Check sheet for the modelled part. Datum: model origin and axes. Units: mm. A direction names the side the tool comes from. Give positions to 0.01 mm unless a question says otherwise; leave off trailing zeros. Write each loop counter-clockwise with the first axis right and the second up, starting at its lowest first coordinate (ties: lowest second). Pieces come first, ordered by that corner, then holes. Notation, with made-up numbers: M 14,47 L 33,47 A11 ccw 33,59 Z; hole C -22,26.25 d10. An arc over 180 degrees is marked long. One line per item, written item: value. Start each with the question number.
Autodesk Inventor part; units mm, degrees
ref_plane "YZ Plane" through (0, 0, 0) normal (1, 0, 0) x (0, 1, 0)
ref_plane "XZ Plane" through (0, 0, 0) normal (0, 1, 0) x (-1, 0, 0)
ref_plane "XY Plane" through (0, 0, 0) normal (0, 0, 1) x (1, 0, 0)
sketch "Boceto1" plane through (0, 0, 0) normal (0, 0, 1) x (1, 0, 0)
  line L0 (3, -11.4) -> (3, -5.5)
  line L1 (3, -5.5) -> (-2.2, -5.5)
  arc A0 (-5.5, -2.2) -> (-2.2, -5.5) centre (-2.2, -2.2) ccw
  line L2 (-5.5, -2.2) -> (-5.5, 2.2)
  arc A1 (-2.2, 5.5) -> (-5.5, 2.2) centre (-2.2, 2.2) ccw
  line L3 (-2.2, 5.5) -> (3, 5.5)
  line L4 (3, 5.5) -> (3, 11.4)
  line L5 (3, 3) -> (-2.2, 3)
  arc A2 (-2.2, 3) -> (-3, 2.2) centre (-2.2, 2.2) ccw
  line L6 (-3, 2.2) -> (-3, -2.2)
  arc A3 (-3, -2.2) -> (-2.2, -3) centre (-2.2, -2.2) ccw
  line L7 (-2.2, -3) -> (3, -3)
  line L8 (3, -3) -> (3, 3)
  line L9 (-2.2, 3.25) -> (3.25, 3.25)
  line L10 (3.25, 3.25) -> (3.25, -3.25)
  line L11 (3.25, -3.25) -> (-2.2, -3.25)
  arc A4 (-3.25, -2.2) -> (-2.2, -3.25) centre (-2.2, -2.2) ccw
  line L12 (-3.25, -2.2) -> (-3.25, 2.2)
  arc A5 (-2.2, 3.25) -> (-3.25, 2.2) centre (-2.2, 2.2) ccw
  line L13 (-2.2, 5) -> (5, 5)
  line L14 (5, 5) -> (5, -5)
  line L15 (5, -5) -> (-2.2, -5)
  arc A6 (-5, -2.2) -> (-2.2, -5) centre (-2.2, -2.2) ccw
  line L16 (-5, -2.2) -> (-5, 2.2)
  arc A7 (-2.2, 5) -> (-5, 2.2) centre (-2.2, 2.2) ccw
  line L17 (5, 0) -> (23, 0)
  line L18 (5, 5) -> (6.5, 5)
  line L19 (8.8007, 5) -> (8.0007, 5)
  line L20 (8.0007, 5) -> (8.0007, -5)
  line L21 (8.0007, -5) -> (8.8007, -5)
  line L22 (8.8007, -5) -> (8.8007, 5)
  line L23 (8.8007, -5) -> (10.3007, -5)
  line L24 (12.6007, -5) -> (11.8007, -5)
  line L25 (11.8007, -5) -> (11.8007, 5)
  line L26 (11.8007, 5) -> (12.6007, 5)
  line L27 (12.6007, 5) -> (12.6007, -5)
  arc A8 (8.8007, -5) -> (11.8007, -5) centre (10.3007, -5) ccw
  arc A9 (8.0007, -5) -> (12.6007, -5) centre (10.3007, -5) ccw
  arc A10 (8.0007, 5) -> (4.9993, 5) centre (6.5, 5) ccw
  arc A11 (8.8007, 5) -> (4.1993, 5) centre (6.5, 5) ccw
  line L28 (16.4021, 5) -> (15.6021, 5)
  line L29 (15.6021, 5) -> (15.6021, -5)
  line L30 (15.6021, -5) -> (16.4021, -5)
  line L31 (16.4021, -5) -> (16.4021, 5)
  line L32 (20.2021, -5) -> (19.4021, -5)
  line L33 (19.4021, -5) -> (19.4021, 5)
  line L34 (19.4021, 5) -> (20.2021, 5)
  line L35 (20.2021, 5) -> (20.2021, -5)
  arc A12 (16.4021, -5) -> (19.4021, -5) centre (17.9021, -5) ccw
  arc A13 (15.6021, -5) -> (20.2021, -5) centre (17.9021, -5) ccw
  arc A14 (15.6021, 5) -> (12.6007, 5) centre (14.1014, 5) ccw
  arc A15 (16.4021, 5) -> (11.8007, 5) centre (14.1014, 5) ccw
  line L36 (24.0036, 5) -> (23.2036, 5)
  line L37 (23.2036, 5) -> (23.2036, -0.2574)
  line L38 (23.2036, -5) -> (24.0036, -5)
  line L39 (24.0036, -1.1409) -> (24.0036, 5)
  arc A16 (23.2036, 5) -> (20.2021, 5) centre (21.7028, 5) ccw
  arc A17 (24.0036, 5) -> (19.4021, 5) centre (21.7028, 5) ccw
  arc A18 (26.3756, 8.5) -> (24.3756, 0) centre (41.5966, 0.4333) ccw
  circle A19 centre (24.3756, 0) radius 1.2
  arc A20 (27.4359, 7.9381) -> (25.5752, 0.0302) centre (41.5966, 0.4333) ccw
  line L40 (25.6, 8.5) -> (25.9736, 8.302)
  arc A21 (27.4359, 7.9381) -> (26.3756, 8.5) centre (26.9058, 8.219) ccw
  arc A22 (24.3756, 0) -> (26.3756, -8.5) centre (41.5966, -0.4333) ccw
  arc A23 (26.3756, -8.5) -> (27.4359, -7.9381) centre (26.9058, -8.219) ccw
  line L41 (26.7492, -8.302) -> (27.4359, -7.9381)
  arc A24 (25.5752, -0.0302) -> (27.4359, -7.9381) centre (41.5966, -0.4333) ccw
  line L42 (23.2036, 0) -> (24.0036, 0)
  point P0 (0, 0)
  point P1 (5, -5)
  point P2 (4.2, -5)
  point P3 (3.8, 5)
  point P4 (25.5036, -5)
  point P5 (22.4, 0)
  point P6 (24.3872, 1.1999)
  point P7 (24.0036, 1.1409)
  point P8 (23.2036, 0.2574)
  point P9 (24.3872, -1.1999)
  point P10 (25.5752, -0.0302)
  point P11 (25.5752, 0.0302)
  dimension "d1" = 0.25
  dimension "d2" = 2
  dimension "d42" = 18
  dimension "d43" = 1.5
  dimension "d45" = 0.8
  dimension "d46" = 10
  dimension "d47" = 1.5
  dimension "d48" = 0.8
  dimension "d49" = 10
  dimension "d50" = 0.8
  dimension "d51" = 10
  dimension "d52" = 1.5
  dimension "d53" = 0.8
  dimension "d54" = 10
  dimension "d55" = 0.8
  dimension "d56" = 10
  dimension "d57" = 1.5
  dimension "d62" = 1.2
extrude "Extrusión1" add sketch "Boceto1" along normal blind 12 contours L13 L14 L15 A6 L16 A7 | A11 L19 A10 L13 | L22 L17 L20 L19 | L22 L21 L20 L17 | L25 L26 L27 L17 | L17 L27 L24 L25 | A8 L24 A9 L21 | A15 L28 A14 L26 | L29 L28 L31 L17 | L17 L31 L30 L29 | L30 A12 L32 A13 | L33 L34 L35 L17 | L17 L35 L32 L33 | A17 L36 A16 L34 | L39 A19 L37 L36 | A19 A18 A22 L39 | L39 L42 L37 A19 | L37 A19 | L39 A19 L37 L42 | A19 A22 A18 | A18 A21 A20 A19 | A19 A24 A23 A22
fillet "Empalme1" radius 0.8 2 edges at (4.1993, 5, 6) (24.3872, -1.1999, 6)
fillet "Empalme1" radius 0.2 2 edges at (24.0036, 1.1409, 6) (24.3872, 1.1999, 6)
properties part number "_3DPrint"
1) Material ranges on L1, parallel to X at y = -6, z = 4.75; L2, parallel to X at y = -6.75, z = 9.25; L3, parallel to X at y = -3.5, z = 3.75, recorded low to high. Write a range as from..to.
2) Tool access check on faces 1 (the flat face through (1, -5, 6)), 2 (the flat face through (8.801, 0, 6)), 3 (the flat face through (15.602, 0, 6)). Record the directions out of +Z, -Z, +X, -X, +Y, -Y that give a thin tool (end or side, any length) a straight path to the whole face; none if there is none.
3) Cross-section at A-A (y = -4). Record the boundary of the cut face in (x, z), plus the area to 3 significant figures.
4) Gauge pin test, flat ends, axial feed: pin 1 (1.6 mm diameter, centred on x = 1.5, z = 5, fed in from +Y); pin 2 (4 mm diameter, centred on y = -5.5, z = 3.5, fed in from -X); pin 3 (1 mm diameter, centred on y = 3.5, z = 6, fed in from +X). Record the tip position at first contact, or that the pin passes through.
5) Cross-section at B-B (x = 21.5). Record the boundary of the cut face in (y, z).
6) Draft check along X on faces 4 (the flat face through (12.601, 0, 6)), 5 (the cylindrical face through (27.175, 8.755, 5.916)), 6 (the flat face through (-5, 0, 6)). Enter one of: released by +X, released by -X, zero draft, split by the parting line, or undercut.
Data:
1. L1: x = 8.23..9.18, 11.42..12.37, 15.83..16.78, 19.02..19.97, 25.29..26.57
1. L2: x = 8.81..11.79, 16.41..19.39, 25.57..26.87
1. L3: x = -4.68..5, 8..8.8, 11.8..12.6, 15.6..16.4, 19.4..20.2, 24.65..25.87
2. face 1: +Z, -Z, -X, -Y
2. face 2: +Z, -Z, +Y
2. face 3: +Z, -Z, -Y
3. outline: M -4.34,0 L 5,0 L 5,12 L -4.34,12 Z; M 8,0 L 8.8,0 L 8.8,12 L 8,12 Z; M 11.8,0 L 12.6,0 L 12.6,12 L 11.8,12 Z; M 15.6,0 L 16.4,0 L 16.4,12 L 15.6,12 Z; M 19.4,0 L 20.2,0 L 20.2,12 L 19.4,12 Z; M 24.74,0 L 25.97,0 L 25.97,12 L 24.74,12 Z
3. area: 165 mm2
4. pin 1: stops at y = 5
4. pin 2: stops at x = -4.68
4. pin 3: stops at x = 25.97
5. outline: M 6.49,0 L 7.29,0 L 7.29,12 L 6.49,12 Z
6. face 4: undercut
6. face 5: split by the parting line
6. face 6: released by -X
